```python
from build123d import *

# Parameters (mm, degrees)
F0_W     = 88.9
F0_H     = 6.35
F1_DEPTH = 43.18
F2_W     = 40.64
F2_H     = 6.35
F3_DEPTH = 41.91
F4_W     = 23.5030670434
F4_H     = 6.35
F4_W_2   = 0.0459178567
F5_DEPTH = 41.91
F6_W     = 23.3165659726
F6_H     = 6.35
F7_DEPTH = 41.91


with BuildPart() as f1:
    # F0 (on Front) → F1 (new body)
    with BuildSketch(Plane.XZ):
        Rectangle(F0_W, F0_H)
    extrude(amount=F1_DEPTH)

    # F2 (on face) → F3 (cut)
    with BuildSketch(Plane(origin=(0, 0, 0), x_dir=(-1, 0, 0), z_dir=(0, 1, 0))):
        Rectangle(F2_W, F2_H)
    extrude(amount=-F3_DEPTH, mode=Mode.SUBTRACT)

    # F4 (on face) → F5 (cut)
    with BuildSketch(Plane.XZ.offset(43.18)):
        with Locations((-32.6984664783, 0)):
            Rectangle(F4_W, F4_H)
        with Locations((-44.4729589283, 0)):
            Rectangle(F4_W_2, F4_H)
    extrude(amount=-F5_DEPTH, mode=Mode.SUBTRACT)

    # F6 (on face) → F7 (cut)
    with BuildSketch(Plane.XZ.offset(43.18)):
        with Locations((32.7917170137, 0)):
            Rectangle(F6_W, F6_H)
    extrude(amount=-F7_DEPTH, mode=Mode.SUBTRACT)


solid = f1.part
```
The listing builds one solid part. Answer for the finished solid, in the listing's coordinates (mm). A direction names the side the tool comes from. Coordinates: 2 decimals unless noted, no trailing zeros. Loops run counter-clockwise (first coordinate to the right, second up) from the corner with the lowest first, then second, coordinate; pieces in that order, holes last. Notation, with made-up numbers: (-33.5, 6.5) - (11.5, 6.5) arc R28 cw to (11.5, 28.5) - close; hole circle Ø7 at (83.25, 22). An arc over 180 degrees is marked (long way). Use a Markdown table: item, result. Add a question column.
1) The mould has two halves that part along X. Classify faces 5 (the flat face through (-20.32, -21, 0)), 6 (the flat face through (33, -1.27, 0)), 7 (the flat face through (-20.947, -23, 0)): released by +X, released by -X, zero draft, split by the parting line, or undercut.
2) For faces 1 (the flat face through (21.133, -23, 0)), 2 (the flat face through (0, -41.91, 0)), 3 (the flat face through (32, 0, 0)), 4 (the flat face through (-33, -1.27, 0)), determine the directions among +Z, -Z, +X, -X, +Y, -Y from which every point of the face is accessible in a straight line to the end or side of a thin tool.
3) The part is cut by section C-C, the plane x = 36. Give the vertices of the cut face in (y, z) (3 decimals), and give its area (3 significant figures).
4) The part is cut by section A-A, the plane y = -40. Give the vertices of the cut face in (x, z) (3 decimals).
5) Given pin 1 (1.9 mm diameter, centred on y = -27, z = -0.5, fed in from -X); pin 2 (3 mm diameter, centred on y = -24.5, z = -0.5, fed in from +X), each flat-ended and moving along its own axis, determine where each tip first touches the part or whether it passes through.
6) Find the intervals of material crossed by line 1 (X direction, y = -34.5, z = 0); line 2 (Y direction, x = 32, z = 0); line 3 (Y direction, x = 1.5, z = 1.75), in increasing order.
7) The part is cut by section B-B, the plane z = -0.75. Give the vertices of the cut face in (x, y), and give its area (3 significant figures).
Here are the results:
| question | item | result |
|---|---|---|
| 1 | face 5 | undercut |
| 1 | face 6 | zero draft |
| 1 | face 7 | released by -X |
| 2 | face 1 | +Z, -Z, +X, -Y |
| 2 | face 2 | +Z, -Z, +Y |
| 2 | face 3 | +Z, -Z, +X, -X, +Y |
| 2 | face 4 | +Z, -Z, -X, -Y |
| 3 | outline | (-1.27, -3.175) - (0, -3.175) - (0, 3.175) - (-1.27, 3.175) - close |
| 3 | area | 8.06 mm^2 |
| 4 | outline | (-20.947, -3.175) - (-20.32, -3.175) - (-20.32, 3.175) - (-20.947, 3.175) - close; (20.32, -3.175) - (21.133, -3.175) - (21.133, 3.175) - (20.32, 3.175) - close |
| 5 | pin 1 | stops at x = -20.95 |
| 5 | pin 2 | stops at x = 21.13 |
| 6 | line 1 | x = -20.95 to -20.32, 20.32 to 21.13 |
| 6 | line 2 | y = -1.27 to 0 |
| 6 | line 3 | y = -43.18 to -41.91 |
| 7 | outline | (-44.45, -1.27) - (-20.95, -1.27) - (-20.95, -43.18) - (21.13, -43.18) - (21.13, -1.27) - (44.45, -1.27) - (44.45, 0) - (20.32, 0) - (20.32, -41.91) - (-20.32, -41.91) - (-20.32, 0) - (-44.45, 0) - close |
| 7 | area | 173 mm^2 |
